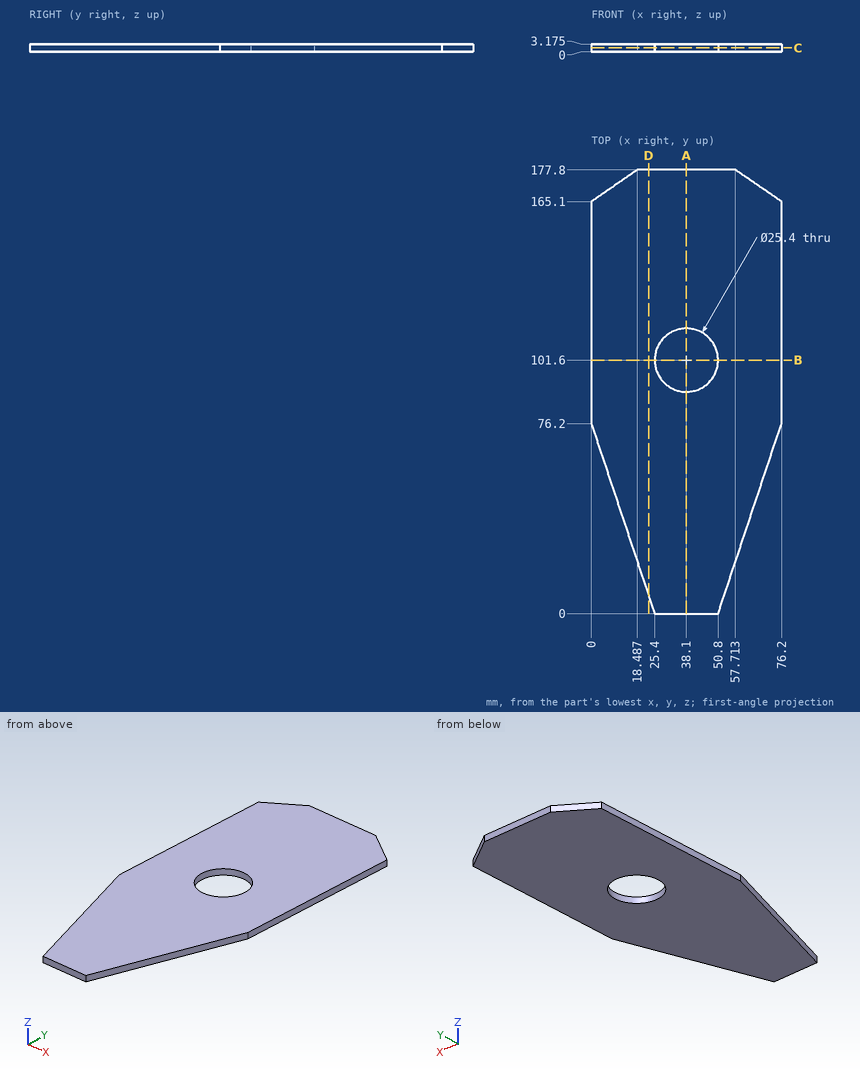
The figure shows three views and two pictorial views of one solid part (mm, origin at its lowest corner). Answer the questions. Give positions to 0.01 mm unless a question says otherwise; leave off trailing zeros. Write each loop counter-clockwise with the first axis right and the second up, starting at its lowest first coordinate (ties: lowest second). Pieces come first, ordered by that corner, then holes. Notation, with made-up numbers: M 32,-40 L 36,-40 A29 cw 36,-8 Z; hole C 43.5,-23 d6. An arc over 180 degrees is marked long. Write each question's results on one line, items separated by ' | '.
Q1. Section C-C, the plane z = 1.6 is taken. Write down the section's boundary in (x, y).
Output values:
outline: M 0,76.2 L 25.4,0 L 50.8,0 L 76.2,76.2 L 76.2,165.1 L 57.71,177.8 L 18.49,177.8 L 0,165.1 Z; hole C 38.1,101.6 d25.4
Q2. Section A-A, the plane x = 38.1 is taken. Write down the section's boundary in (y, z) (1 decimal).
Output values:
outline: M 0,0 L 88.9,0 L 88.9,3.2 L 0,3.2 Z; M 114.3,0 L 177.8,0 L 177.8,3.2 L 114.3,3.2 Z
Q3. Section B-B, the plane y = 101.6 is taken. Write down the section's boundary in (x, z) (1 decimal).
Output values:
outline: M 0,0 L 25.4,0 L 25.4,3.2 L 0,3.2 Z; M 50.8,0 L 76.2,0 L 76.2,3.2 L 50.8,3.2 Z
Q4. Flat-ended cylindrical pins translate along their axes: P1, Ø20.5, axis at x = 38.1, y = 101.6, coming from the -Z side; P2, Ø1.5, axis at y = 39.5, z = 1.5, coming from the -X side. Find the tip coordinate at first contact, or state that the pin passes through.
Output values:
P1: through | P2: x = 11.98
Q5. Consider L1, parallel to Y at x = 38.1, z = 0.7; L2, parallel to Y at x = 33.5, z = 1.4; L3, parallel to X at y = 91, z = 2.9 (1 decimal). Determine where each line is inside the solid, lowest interval first. Write a range as from..to.
Output values:
L1: 0..88.9, 114.3..177.8 | L2: 0..89.76, 113.44..177.8 | L3: 0..31.1, 45.1..76.2
Q6. Section D-D, the plane x = 23 is taken. Write down the section's boundary in (y, z) (1 decimal).
Output values:
outline: M 7.2,0 L 177.8,0 L 177.8,3.2 L 7.2,3.2 Z
